Can you work these out from the model? Positions are in its coordinate system, mm. Face numbers are marked on the shaded views. Give positions to 0.01 mm unless a question says otherwise; leave off trailing zeros. Write each loop counter-clockwise with the first axis right and the second up, starting at its lowest first coordinate (ties: lowest second). Pieces come first, ordered by that corner, then holes. Notation, with made-up numbers: (4.5, 10.5) -> (42.5, 10.5) arc R21 ccw to (42.5, 39.5) -> close; hole circle Ø6 at (40, -17). An arc over 180 degrees is marked (long way). One line per item, written item: value.
from build123d import *

# Parameters (mm, degrees)
F0_R     = 3.81
F0_R_2   = 15.875
F1_DEPTH = 19.05
F2_DEPTH = 31.369
F3_R     = 7.62
F4_R     = 7.62


with BuildPart() as f1:
    # F0 (on Front) → F1 (new body)
    with BuildSketch(Plane.XZ):
        Polygon((-69.850003, -88.899992), (69.849997, -88.900008), (69.850003, 88.899992), (0, 158.75), (-69.849997, 88.900008), align=None)
        with Locations((0, 12.7)):
            Circle(F0_R, mode=Mode.SUBTRACT)
        with Locations((0, 44.45)):
            Circle(F0_R_2, mode=Mode.SUBTRACT)
    extrude(amount=F1_DEPTH)

    # F0 (on Front) → F2 (join, symmetric)
    with BuildSketch(Plane.XZ):
        with Locations((0, 12.7)):
            Circle(F0_R)
    extrude(amount=F2_DEPTH, both=True)

    # F3
    f3_edges = [f1.edges().sort_by_distance(p)[0] for p in [
        (69.85, 0, -8e-06),
    ]]
    fillet(f3_edges, radius=F3_R)

    # F4
    f4_edges = [f1.edges().sort_by_distance(p)[0] for p in [
        (-69.85, 0, 8e-06),
    ]]
    fillet(f4_edges, radius=F4_R)


solid = f1.part
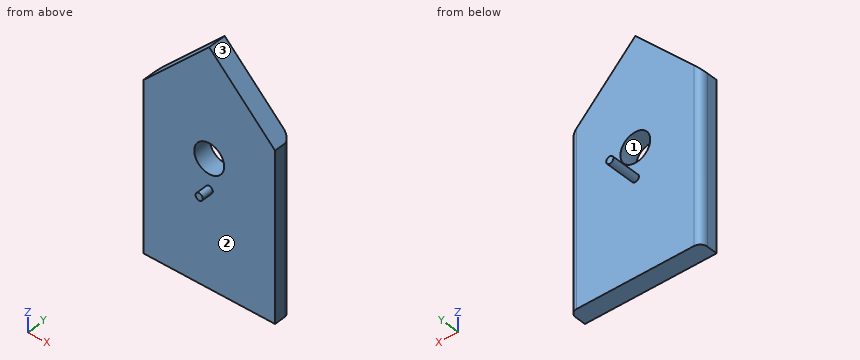
1) If we section it at B-B (x = 27): Write out the boundary of the cut face in (y, z), and give its area (3 significant figures).
Answer list:
outline: (-19.05, -88.9) -> (0, -88.9) -> (0, 131.75) -> (-19.05, 131.75) -> close
area: 4,200 mm^2
2) Will these pins go through, and if not, where does the flat tip stop? pin 1 (4 mm diameter, centred on x = 21, z = 112, fed in from +Y); pin 2 (6 mm diameter, centred on x = -3.5, y = 17.5, fed in from +Z); pin 3 (12 mm diameter, centred on x = -31.5, z = -63, fed in from -Y).
Answer list:
pin 1: stops at y = 0
pin 2: stops at z = 16.48
pin 3: stops at y = -19.05
3) If we section it at A-A (z = 44.45): Write out the boundary of the cut face in (x, y) (3 decimals).
Answer list:
outline: (-69.85, -19.05) -> (-15.875, -19.05) -> (-15.875, 0) -> (-62.23, 0) arc R7.62 ccw to (-69.85, -7.62) -> close; (15.875, -19.05) -> (69.85, -19.05) -> (69.85, -7.62) arc R7.62 ccw to (62.23, 0) -> (15.875, 0) -> close
4) If we section it at C-C (z = 12.7): Write out the boundary of the cut face in (x, y), and give its area (3 significant figures).
Answer list:
outline: (-69.85, -19.05) -> (-3.81, -19.05) -> (-3.81, -31.37) -> (3.81, -31.37) -> (3.81, -19.05) -> (69.85, -19.05) -> (69.85, -7.62) arc R7.62 ccw to (62.23, 0) -> (3.81, 0) -> (3.81, 31.37) -> (-3.81, 31.37) -> (-3.81, 0) -> (-62.23, 0) arc R7.62 ccw to (-69.85, -7.62) -> close
area: 2,970 mm^2
5) I need wall thicknesses on L1, parallel to X at y = -14, z = 44; L2, parallel to Z at x = 0, y = -4 (3 decimals); L3, parallel to Y at x = 44, z = 12.5. Which ranges of each line are inside material? Lowest first, please.
Answer list:
L1: x = -69.85 to -15.87, 15.87 to 69.85
L2: z = -88.9 to 28.575, 60.325 to 158.75
L3: y = -19.05 to 0
6) If we section it at D-D (y = -2.5): Write out the boundary of the cut face in (x, z) (3 decimals), and give its area (3 significant figures).
Answer list:
outline: (-67.874, -88.9) -> (67.874, -88.9) -> (67.874, 90.876) -> (0, 158.75) -> (-67.874, 90.876) -> close; hole circle Ø31.75 at (0, 44.45)
area: 28,200 mm^2
7) We'd pull the mould along Z, two halves only. Please class the marked faces 1, 2 and 3: released by +Z, released by -Z, zero draft, split by the parting line, or undercut.
Answer list:
face 1: undercut
face 2: zero draft
face 3: released by +Z
